Autodesk Inventor part; units mm, degrees
ref_plane "YZ Plane" through (0, 0, 0) normal (1, 0, 0) x (0, 1, 0)
ref_plane "XZ Plane" through (0, 0, 0) normal (0, 1, 0) x (-1, 0, 0)
ref_plane "XY Plane" through (0, 0, 0) normal (0, 0, 1) x (1, 0, 0)
sketch "Эскиз1" plane through (0, 0, 0) normal (0, 0, 1) x (1, 0, 0)
  circle A0 centre (0, 0) radius 3
  circle A1 centre (0, 0) radius 4
  dimension "d0" = 6
  dimension "d1" = 8
extrude "Выдавливание1" add sketch "Эскиз1" along normal blind 10
sketch "Эскиз2" plane through (0, 0, 10) normal (0, 0, 1) x (1, 0, 0)
  circle A0 centre (0, 0) radius 5
  circle A1 centre (0, 0) radius 4
  dimension "d4" = 10
extrude "Выдавливание2" add sketch "Эскиз2" against normal blind 2
fillet "Сопряжение1" radius 2 1 edges at (-5, 0, 10)
properties part number "hole_small" material "Латунь"
Model file for the job. Use its own axes, mm. Round coordinates to 2 decimals unless told otherwise and drop trailing zeros. Order: outer loops, then holes, each group sorted by start corner. A loop starts at its lowest first (then second) coordinate and runs counter-clockwise, first axis right, second up. Notation, with made-up numbers: (6.5, 89) -> (30.5, 89) arc R34 ccw to (30.5, 128) -> close; hole circle Ø9 at (54, -40). An arc over 180 degrees is marked (long way). Use one line per item in the form item = value.
Item 1: Pull direction X, two halves, no side cores. Call faces 1 (the face through (1, 3, 0)), 2 (the face through (-3, 0, 5)), 3 (the face through (-0.867, 3.905, 3.944)): released by +X, released by -X, zero draft, split by the parting line, or undercut.
Returned:
face_1 = zero draft
face_2 = undercut
face_3 = split by the parting line
Item 2: Drill centre lines: line 1 (Y direction, x = 0, z = 3.75); line 2 (X direction, y = -1, z = 4.5); line 3 (X direction, y = 2, z = 2.5). Where is each one in solid material? Low to high.
Returned:
line_1 = -4 to -3, 3 to 4
line_2 = -3.87 to -2.83, 2.83 to 3.87
line_3 = -3.46 to -2.24, 2.24 to 3.46
Item 3: Cut at C-C, the plane z = 4. Write the cut outline in (x, y), and give its area (3 significant figures).
Returned:
outline = circle Ø8 at (0, 0); hole circle Ø6 at (0, 0)
area = 22.0 mm^2
Item 4: Flat gauge pins, fed straight in: pin 1 Ø2 at (x, z) = (1.5, 4.5) entering from -Y; pin 2 Ø2 at (x, z) = (-3.5, 5.5) entering from -Y; pin 3 Ø2 at (x, z) = (-2, 4.5) entering from -Y. Where does each tip first touch, or does it go through?
Returned:
pin_1 = -3.97
pin_2 = -3.12
pin_3 = -3.87
Item 5: Cut at D-D, the plane z = 8.5. Write the cut outline in (x, y), and give its area (3 significant figures).
Returned:
outline = circle Ø9.87 at (0, 0); hole circle Ø6 at (0, 0)
area = 48.3 mm^2
